Autodesk Inventor part; units mm, degrees
ref_plane "YZ Plane" through (0, 0, 0) normal (1, 0, 0) x (0, 1, 0)
ref_plane "XZ Plane" through (0, 0, 0) normal (0, 1, 0) x (-1, 0, 0)
ref_plane "XY Plane" through (0, 0, 0) normal (0, 0, 1) x (1, 0, 0)
sketch "Skizze1" plane through (0, 0, 0) normal (0, 1, 0) x (-1, 0, 0)
  line L0 (0, 0) -> (-129.5, 0)
  line L1 (-129.5, 0) -> (-129.5, -51.5)
  line L2 (-129.5, -51.5) -> (0, -51.5)
  line L3 (0, -51.5) -> (0, 0)
  line L4 (-122, 0) -> (-122, -15)
  line L5 (-122, -15) -> (-105.5, -15)
  line L6 (-105.5, -15) -> (-105.5, 0)
  dimension "d0" = 129.5
  dimension "d1" = 51.5
  dimension "d4" = 16.5
  dimension "d5" = 7.5
  dimension "d6" = 15
extrude "Extrusion1" add sketch "Skizze1" along normal blind 3 contours L3 L2 L1 L0 L4 L5 L6
sketch "Skizze2" plane through (0, 3, 0) normal (0, 1, 0) x (1, 0, 0)
  line L0 (10, 45) -> (79.5, 45) construction
  line L1 (10, 43.5) -> (79.5, 43.5)
  line L2 (79.5, 46.5) -> (10, 46.5)
  arc A0 (10, 46.5) -> (10, 43.5) centre (10, 45) ccw
  arc A1 (79.5, 43.5) -> (79.5, 46.5) centre (79.5, 45) ccw
  line L3 (0, 0) -> (105.5, 0)
  line L4 (105.5, 0) -> (105.5, 15)
  line L5 (105.5, 15) -> (122, 15)
  line L6 (122, 15) -> (122, 0)
  line L7 (122, 0) -> (129.5, 0)
  line L8 (129.5, 0) -> (129.5, 51.5)
  line L9 (129.5, 51.5) -> (0, 51.5)
  line L10 (0, 51.5) -> (0, 0)
  point P0 (44.75, 45)
  dimension "d7" = 5
  dimension "d8" = 10
  dimension "d9" = 50
  dimension "d10" = 1.5
extrude "Extrusion2" cut sketch "Skizze2" against normal through all contours A0 L2 A1 L1
pattern_linear "Rechteckige Anordnung1" count 5 spacing 5 along (0, 0, 1) of "Extrusion2"
properties part number "wood_front"
Source: CAD feature listing. Evaluate the final solid. Frame: model axes, mm. A direction names the side the tool comes from. Round coordinates to 2 decimals unless told otherwise and drop trailing zeros. Order: outer loops, then holes, each group sorted by start corner. A loop starts at its lowest first (then second) coordinate and runs counter-clockwise, first axis right, second up. Notation, with made-up numbers: (17, -4.5) - (26, -4.5) arc R11 cw to (26, 2.5) - close; hole circle Ø4 at (44.5, 87.5). An arc over 180 degrees is marked (long way). Use a Markdown table: item, result. Add a question column.
1. Set-up query: faces 3 (the flat face through (105.5, 1, -8)), 4 (the flat face through (45, 2, -41.5)). Return all of +Z, -Z, +X, -X, +Y, -Y with unobstructed straight access to the full face (end or side cutting, diameter ignored); none if empty.
2. First-contact query: pin 1 (1.5 mm diameter, centred on x = 112, y = 1.5, fed in from +Z). Flat tip, straight axial feed; report the tip coordinate or a pass-through.
3. Section query D-D (z = -45). Return the cut outline in (x, y), then the cut area to 3 significant figures.
4. Mould query, pull axis X, two halves, no side actions, for faces 1 (the flat face through (129.5, 1, -25)), 2 (the cylindrical face through (8.5, 1.5, -25)). Classes: +X half, -X half, draft (parallel to the pull), parting line (faces both ways), or undercut.
5. Section query C-C (y = 0.9). Return the cut outline in (x, z), then the cut area to 3 significant figures.
6. Section query A-A (z = -5). Return the cut outline in (x, y).
7. Line query: probe 1 along Z at (x, y) = (47.5, 2.2); probe 2 along X at (y, z) = (0.4, -13.5); probe 3 along X at (y, z) = (1.4, -40). Output: solid intervals per line, ascending.
8. Section query B-B (x = 59). Return the cut outline in (y, z).
Derived:
| question | item | result |
|---|---|---|
| 1 | face 3 | +Z, +Y, -Y |
| 1 | face 4 | +Y, -Y |
| 2 | pin 1 | z = -15 |
| 3 | outline | (0, 0) - (8.5, 0) - (8.5, 3) - (0, 3) - close; (81, 0) - (129.5, 0) - (129.5, 3) - (81, 3) - close |
| 3 | area | 171 mm2 |
| 4 | face 1 | +X half |
| 4 | face 2 | undercut |
| 5 | outline | (0, -51.5) - (129.5, -51.5) - (129.5, 0) - (122, 0) - (122, -15) - (105.5, -15) - (105.5, 0) - (0, 0) - close; hole (10, -46.5) - (79.5, -46.5) arc R1.5 ccw to (79.5, -43.5) - (10, -43.5) arc R1.5 ccw to start; hole (10, -41.5) - (79.5, -41.5) arc R1.5 ccw to (79.5, -38.5) - (10, -38.5) arc R1.5 ccw to start; hole (10, -36.5) - (79.5, -36.5) arc R1.5 ccw to (79.5, -33.5) - (10, -33.5) arc R1.5 ccw to start; hole (10, -31.5) - (79.5, -31.5) arc R1.5 ccw to (79.5, -28.5) - (10, -28.5) arc R1.5 ccw to start; hole (10, -26.5) - (79.5, -26.5) arc R1.5 ccw to (79.5, -23.5) - (10, -23.5) arc R1.5 ccw to start |
| 5 | area | 5,340 mm2 |
| 6 | outline | (0, 0) - (105.5, 0) - (105.5, 3) - (0, 3) - close; (122, 0) - (129.5, 0) - (129.5, 3) - (122, 3) - close |
| 7 | probe 1 | -51.5 to -46.5, -43.5 to -41.5, -38.5 to -36.5, -33.5 to -31.5, -28.5 to -26.5, -23.5 to 0 |
| 7 | probe 2 | 0 to 105.5, 122 to 129.5 |
| 7 | probe 3 | 0 to 8.5, 81 to 129.5 |
| 8 | outline | (0, -51.5) - (3, -51.5) - (3, -46.5) - (0, -46.5) - close; (0, -43.5) - (3, -43.5) - (3, -41.5) - (0, -41.5) - close; (0, -38.5) - (3, -38.5) - (3, -36.5) - (0, -36.5) - close; (0, -33.5) - (3, -33.5) - (3, -31.5) - (0, -31.5) - close; (0, -28.5) - (3, -28.5) - (3, -26.5) - (0, -26.5) - close; (0, -23.5) - (3, -23.5) - (3, 0) - (0, 0) - close |
